from build123d import *

# Parameters (mm, degrees)
BOSS_EXTRUDE1_START = 6
SKETCH2_R           = 10
SKETCH2_R_2         = 2.5
BOSS_EXTRUDE1_DEPTH = 6
SKETCH3_W           = 5.7
SKETCH3_H           = 2.7
CUT_EXTRUDE1_DEPTH  = 5
SKETCH4_R           = 1.65
CUT_EXTRUDE2_DEPTH  = 35


with BuildPart() as part:
    # Sketch1 → Revolve1 (revolve)
    with BuildSketch(Plane.XY, mode=Mode.PRIVATE) as revolve1_sk:
        Polygon((2.5, 8), (15, 8), (15, 4.4), (14.6, 4), (15, 3.6), (15, 0), (2.5, 0), align=None)
    revolve(revolve1_sk.sketch.rotate(Axis((0, 0, 0), (0, 1, 0)), 90), axis=Axis((0, 0, 0), (0, 1, 0)))

    # Sketch2 → Boss-Extrude1 (add)
    with BuildSketch(Plane(origin=(0, 8, 0), x_dir=(1, 0, 0), z_dir=(0, 1, 0)).offset(BOSS_EXTRUDE1_START)):
        with Locations(Location((0, 0, 0), (0, 0, 270))):
            Circle(SKETCH2_R)
        with Locations(Location((0, 0, 0), (0, 0, 90))):
            Circle(SKETCH2_R_2, mode=Mode.SUBTRACT)
    extrude(amount=-BOSS_EXTRUDE1_DEPTH)

    # Sketch3 → Cut-Extrude1 (cut)
    with BuildSketch(Plane(origin=(0, 14, 0), x_dir=(1, 0, 0), z_dir=(0, 1, 0))):
        with Locations((0, -7)):
            Rectangle(SKETCH3_W, SKETCH3_H)
    extrude(amount=-CUT_EXTRUDE1_DEPTH, mode=Mode.SUBTRACT)

    # Sketch4 → Cut-Extrude2 (cut)
    with BuildSketch(Plane.XY):
        with Locations(Location((0, 11, 0), (0, 0, 180))):
            Circle(SKETCH4_R)
    extrude(amount=CUT_EXTRUDE2_DEPTH, mode=Mode.SUBTRACT)


solid = part.part
Can you work these out from the model? Positions are in its coordinate system, mm. A direction names the side the tool comes from. Give positions to 0.01 mm unless a question says otherwise; leave off trailing zeros. Order: outer loops, then holes, each group sorted by start corner. A loop starts at its lowest first (then second) coordinate and runs counter-clockwise, first axis right, second up. Notation, with made-up numbers: M 60,8.25 L 98,8.25 A28 cw 98,34.25 Z; hole C -19,56.25 d5. An arc over 180 degrees is marked long. Use a Markdown table: item, result. Add a question column.
Item 1: We'd pull the mould along Y, two halves only. Please class faces 1 (the flat face through (0, 9, 7)), 2 (the cylindrical face through (1.65, 10.93, 9.16)), 3 (the flat face through (2.85, 12, 7)): +Y half, -Y half, draft (parallel to the pull), parting line (faces both ways), or undercut.
Item 2: Will these pins go through, and if not, where does the flat tip stop? pin 1 (1 mm diameter, centred on y = 6.5, z = -2.5, fed in from +X); pin 2 (1 mm diameter, centred on y = 7, z = -11, fed in from +X); pin 3 (2 mm diameter, centred on x = 1.5, y = 3.5, fed in from -Z); pin 4 (3 mm diameter, centred on x = 0, z = 0, fed in from -Y).
Item 3: Suppose I cut it at D-D (y = 11). List the corners of the cut face in (x, z) for me.
Item 4: If I drill on L1, parallel to Y at x = 0, z = 9.4; L2, parallel to X at y = 6.75, z = 0; L3, parallel to Y at x = 5.5, z = -10, over which ranges is the centre line in solid material (lowest first)? Write a range as [from, to].
Item 5: For faces 4 (the flat face through (-1, 13, 8.35)), 5 (the flat face through (-2, 14, -2)), 6 (the cylindrical face through (-0.761, 12.464, 3.738)), which set-ups out of +Z, -Z, +X, -X, +Y, -Y let a thin tool reach every point of the face, with its end or its side?
Item 6: Suppose I cut it at C-C (y = 7.5). List the corners of the cut face in (x, z) for me, then the cut area to 3 significant figures.
Item 7: Suppose I cut it at A-A (x = 0). Count the separate pieces of the cut face and the enclosed holes in it, then the cut area to 3 significant figures.
Item 8: Suppose I cut it at B-B (z = 0). List the corners of the cut face in (x, y) for me, then the cut area to 3 significant figures.
Answer sheet:
| question | item | result |
|---|---|---|
| 1 | face 1 | +Y half |
| 1 | face 2 | undercut |
| 1 | face 3 | draft |
| 2 | pin 1 | stops at x = 14.87 |
| 2 | pin 2 | stops at x = 10.71 |
| 2 | pin 3 | stops at z = -14.99 |
| 2 | pin 4 | passes through |
| 3 | outline | M -2.85,5.65 L -2.85,8.35 L -1.65,8.35 L -1.65,9.86 A10 ccw long 1.65,9.86 L 1.65,8.35 L 2.85,8.35 L 2.85,5.65 L 1.65,5.65 L 1.65,1.88 A2.5 cw long -1.65,1.88 L -1.65,5.65 Z |
| 4 | L1 | y = [0, 9.35], [12.65, 14] |
| 4 | L2 | x = [-15, -2.5], [2.5, 15] |
| 4 | L3 | y = [0, 8] |
| 5 | face 4 | +Y |
| 5 | face 5 | +Z, -Z, +X, -X, +Y |
| 5 | face 6 | +Z |
| 6 | outline | C 0,0 d30; hole C 0,0 d5 |
| 6 | area | 687 mm² |
| 7 | separate pieces | 4 |
| 7 | enclosed holes | 0 |
| 7 | area | 260 mm² |
| 8 | outline | M -15,0 L -2.5,0 L -2.5,14 L -10,14 L -10,8 L -15,8 L -15,4.4 L -14.6,4 L -15,3.6 Z; M 2.5,0 L 15,0 L 15,3.6 L 14.6,4 L 15,4.4 L 15,8 L 10,8 L 10,14 L 2.5,14 Z |
| 8 | area | 290 mm² |
